Could you check a few things on this model? Use its own coordinates, in mm. A direction names the side the tool comes from. Give positions to 0.01 mm unless a question says otherwise; leave off trailing zeros. Write each loop counter-clockwise with the first axis right and the second up, starting at its lowest first coordinate (ties: lowest second). Pieces come first, ordered by that corner, then holes. Notation, with made-up numbers: M 25.5,58 L 46.5,58 A26 ccw 46.5,72 Z; hole C 35,-5 d7. An arc over 180 degrees is marked long. Use one line per item in the form item = value.
from build123d import *

# Parameters (mm, degrees)
CHAMFER1_SIZE      = 0.5
CHAMFER2_SIZE      = 0.3
CUT_EXTRUDE1_DEPTH = 2.5
CHAMFER3_SIZE      = 0.3


with BuildPart() as part:
    # Sketch1 → Revolve1 (revolve)
    with BuildSketch(Plane.XY):
        Polygon((0, 0), (0, 2.75), (3, 2.75), (3, 1.49), (9, 1.49), (9, 0), align=None)
    revolve(axis=Axis((-88.705490849, 0, 0), (1, 0, 0)))

    # Chamfer1
    chamfer1_edges = [part.edges().sort_by_distance(p)[0] for p in [
        (9, -1.49, 0),
    ]]
    chamfer(chamfer1_edges, length=CHAMFER1_SIZE)

    # Chamfer2
    chamfer2_edges = [part.edges().sort_by_distance(p)[0] for p in [
        (0, -2.75, 0),
    ]]
    chamfer(chamfer2_edges, length=CHAMFER2_SIZE)

    # Sketch3 → Cut-Extrude1 (cut)
    with BuildSketch(Plane(origin=(0, 0, 0), x_dir=(0, 0, -1), z_dir=(1, 0, 0))):
        Polygon((-1.443375673, 0), (-0.721687836, -1.25), (0.721687836, -1.25), (1.443375673, 0), (0.721687836, 1.25), (-0.721687836, 1.25), align=None)
    extrude(amount=CUT_EXTRUDE1_DEPTH, mode=Mode.SUBTRACT)

    # Chamfer3
    chamfer3_edges = [part.edges().sort_by_distance(p)[0] for p in [
        (0, 0.625, 1.082531755),
        (0, -0.625, 1.082531755),
        (0, -1.25, 0),
        (0, -0.625, -1.082531755),
        (0, 0.625, -1.082531755),
        (0, 1.25, 0),
    ]]
    chamfer(chamfer3_edges, length=CHAMFER3_SIZE)


solid = part.part
1) I want a section at A-A, the plane x = 2.25. Please give me the cut outline in (y, z), plus the area to 3 significant figures.
Checked values:
outline = C 0,0 d5.5; hole M -1.25,-0.72 L 0,-1.44 L 1.25,-0.72 L 1.25,0.72 L 0,1.44 L -1.25,0.72 Z
area = 18.3 mm2
2) For faces 1 (the flat face through (1, 1.25, 0)), 2 (the flat face through (9, 0, 0)), 3 (the cylindrical face through (5.788, -0.194, 1.477)), which set-ups out of +Z, -Z, +X, -X, +Y, -Y let a thin tool reach every point of the face, with its end or its side?
Checked values:
face_1 = -X
face_2 = +Z, -Z, +X, +Y, -Y
face_3 = +X
3) If I drill on L1, parallel to Z at x = 2, y = 2.45; L2, parallel to X at y = 1.5, z = -1.05; L3, parallel to Y at x = 2.25, z = 0.9, over which ranges is the centre line in solid material (lowest first)?
Checked values:
L1 = -1.25 to 1.25
L2 = 0 to 3
L3 = -2.6 to -0.94, 0.94 to 2.6
4) I want a section at C-C, the plane x = 3.75. Please give me the cut outline in (y, z), plus the area to 3 significant figures.
Checked values:
outline = C 0,0 d2.98
area = 6.97 mm2
5) I want a section at B-B, the plane z = 0. Please give me the cut outline in (x, y).
Checked values:
outline = M 0,-2.45 L 0.3,-2.75 L 3,-2.75 L 3,-1.49 L 8.5,-1.49 L 9,-0.99 L 9,0.99 L 8.5,1.49 L 3,1.49 L 3,2.75 L 0.3,2.75 L 0,2.45 L 0,1.55 L 0.3,1.25 L 2.5,1.25 L 2.5,-1.25 L 0.3,-1.25 L 0,-1.55 Z
6) Thinking about a two-plate mould opening in Z: for faces 4 (the flat face through (0.15, -0.69, 1.22)), 5 (the cylindrical face through (1.669, -0.596, -2.685)), 6 (the flat face through (3, 1.2, -1.2)), which applies, released by +Z, released by -Z, zero draft, split by the parting line, or undercut?
Checked values:
face_4 = undercut
face_5 = split by the parting line
face_6 = zero draft
7) For pin 1 Ø1 at (y, z) = (-1.5, 2) entering from +X; pin 2 Ø1.5 at (y, z) = (0.5, -1.5) entering from +X; pin 3 Ø1 at (x, z) = (6, -0.5) entering from +Y; pin 4 Ø1.5 at (x, z) = (8, -1) entering from -Y, each with a flat end and sliding along its axis, tell me the tip position at first contact or that it passes through.
Checked values:
pin_1 = 3
pin_2 = 9
pin_3 = 1.49
pin_4 = -1.47
